Design review of the part built by this model. Coordinates are the model's own, in mm. Round coordinates to 2 decimals unless told otherwise and drop trailing zeros. Write each loop counter-clockwise with the first axis right and the second up, starting at its lowest first coordinate (ties: lowest second). Pieces come first, ordered by that corner, then holes.
from build123d import *

# Parameters (mm, degrees)
SKETCH1_W           = 6
SKETCH1_H           = 50
SKETCH1_W_2         = 50
SKETCH1_H_2         = 6
BOSS_EXTRUDE1_DEPTH = 6


with BuildPart() as part:
    # Sketch1 → Boss-Extrude1 (new body)
    with BuildSketch(Plane(origin=(0, 0, 0), x_dir=(0, 0, -1), z_dir=(1, 0, 0))):
        with BuildLine():
            Line((-414.831767264, 67.151199882), (3.168232736, 67.151199882))
            ThreePointArc((3.168232736, 67.151199882), (73.878910855, 37.861878001), (103.168232736, -32.848800118))
            Line((103.168232736, -32.848800118), (103.168232736, -336.848800118))
            Line((103.168232736, -336.848800118), (-414.831767264, -336.848800118))
            Line((-414.831767264, -336.848800118), (-414.831767264, 67.151199882))
        make_face()
        with Locations((-393.831767264, -7.848800118)):
            Rectangle(SKETCH1_W, SKETCH1_H, mode=Mode.SUBTRACT)
        with Locations((-393.831767264, -261.848800118)):
            Rectangle(SKETCH1_W, SKETCH1_H, mode=Mode.SUBTRACT)
        with Locations((-253.831767264, -315.848800118)):
            Rectangle(SKETCH1_W_2, SKETCH1_H_2, mode=Mode.SUBTRACT)
        with Locations((-57.831767264, -315.848800118)):
            Rectangle(SKETCH1_W_2, SKETCH1_H_2, mode=Mode.SUBTRACT)
        with Locations((-253.831767264, -225.848800118)):
            Rectangle(SKETCH1_W_2, SKETCH1_H_2, mode=Mode.SUBTRACT)
        with Locations((-57.831767264, -225.848800118)):
            Rectangle(SKETCH1_W_2, SKETCH1_H_2, mode=Mode.SUBTRACT)
        with Locations((-253.831767264, -135.848800118)):
            Rectangle(SKETCH1_W_2, SKETCH1_H_2, mode=Mode.SUBTRACT)
        with Locations((-57.831767264, -135.848800118)):
            Rectangle(SKETCH1_W_2, SKETCH1_H_2, mode=Mode.SUBTRACT)
        with Locations((-253.831767264, -45.848800118)):
            Rectangle(SKETCH1_W_2, SKETCH1_H_2, mode=Mode.SUBTRACT)
        with Locations((-57.831767264, -45.848800118)):
            Rectangle(SKETCH1_W_2, SKETCH1_H_2, mode=Mode.SUBTRACT)
    extrude(amount=BOSS_EXTRUDE1_DEPTH)


solid = part.part
1) For P1, Ø6, axis at y = -68, z = 206.5, coming from the -X side, flat-tipped, find the tip position at first contact; note if it passes through.
2) For line 1 along Y through (x, z) = (3.2, 66); line 2 along Z through (x, y) = (4.1, -134); line 3 along Z through (x, y) = (4.5, 1.5), list the stretches that pass through material, from the lowest coordinate up.
3) Add section A-A on y = -12.5. State the section outline as (x, z) points.
4) Add section C-C on y = 35. State the section outline as (x, z) points, and give its area (3 significant figures).
5) Add section B-B on x = 4.5. Count the separate pieces of the cut face and the enclosed holes in it, and give its area (3 significant figures).
Computed:
1. P1: stops at x = 0
2. line 1: y = -336.85 to -318.85, -312.85 to -228.85, -222.85 to -138.85, -132.85 to -48.85, -42.85 to 67.15
2. line 2: z = -103.17 to 32.83, 82.83 to 228.83, 278.83 to 414.83
2. line 3: z = -97.08 to 390.83, 396.83 to 414.83
3. outline: (0, -101.08) - (6, -101.08) - (6, 390.83) - (0, 390.83) - close; (0, 396.83) - (6, 396.83) - (6, 414.83) - (0, 414.83) - close
4. outline: (0, -76.63) - (6, -76.63) - (6, 414.83) - (0, 414.83) - close
4. area: 2,950 mm2
5. separate pieces: 1
5. enclosed holes: 10
5. area: 204,000 mm2
